Could you check a few things on this model? Use its own coordinates, in mm. Face numbers are marked on the shaded views. A direction names the side the tool comes from. Round coordinates to 2 decimals unless told otherwise and drop trailing zeros. Loops run counter-clockwise (first coordinate to the right, second up) from the corner with the lowest first, then second, coordinate; pieces in that order, holes last. Notation, with made-up numbers: (8, 71.25) -> (35, 71.25) arc R24 cw to (35, 101.25) -> close; hole circle Ø10 at (20.25, 55). An arc over 180 degrees is marked (long way). One line per item, written item: value.
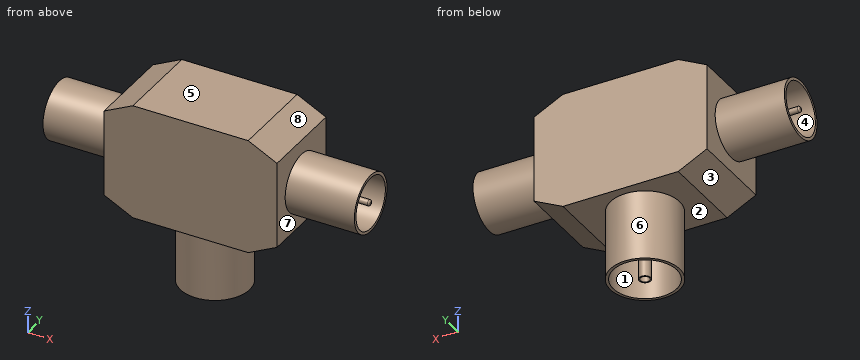
from build123d import *

# Parameters (mm, degrees)
BOSS_EXTRUDE1_DEPTH  = 15
SKETCH2_R            = 6
SKETCH2_R_2          = 5.5
BOSS_EXTRUDE2_DEPTH  = 12
SKETCH3_R            = 1
SKETCH3_R_2          = 0.8
BOSS_EXTRUDE3_DEPTH  = 12
SKETCH4_R            = 5
SKETCH4_R_2          = 4.5
SKETCH4_R_3          = 0.5
BOSS_EXTRUDE4_DEPTH  = 12
FILLET2_R            = 0.3
FILLET2_OF_MIRROR1_R = 0.3


with BuildPart() as part:
    # Sketch1 → Boss-Extrude1 (new body)
    with BuildSketch(Plane(origin=(0, 0, 0), x_dir=(1, 0, 0), z_dir=(0, 1, 0))):
        Polygon((10, 20), (15, 17.5), (15, 2.5), (10, 0), (-10, 0), (-15, 2.5), (-15, 17.5), (-10, 20), align=None)
    extrude(amount=BOSS_EXTRUDE1_DEPTH)

    # Sketch2 → Boss-Extrude2 (add)
    with BuildSketch(Plane(origin=(0, 0, -20), x_dir=(-1, 0, 0), z_dir=(0, 0, -1))):
        with Locations((0, 7.5)):
            Circle(SKETCH2_R)
        with Locations((0, 7.5)):
            Circle(SKETCH2_R_2, mode=Mode.SUBTRACT)
    extrude(amount=BOSS_EXTRUDE2_DEPTH)

    # Sketch3 → Boss-Extrude3 (add)
    with BuildSketch(Plane(origin=(0, 0, -20), x_dir=(-1, 0, 0), z_dir=(0, 0, -1))):
        with Locations((0, 7.5)):
            Circle(SKETCH3_R)
        with Locations((0, 7.5)):
            Circle(SKETCH3_R_2, mode=Mode.SUBTRACT)
    extrude(amount=BOSS_EXTRUDE3_DEPTH)

    # Sketch4 → Boss-Extrude4 (add)
    with BuildSketch(Plane.ZY.offset(15)):
        with Locations((-10, 7.5)):
            Circle(SKETCH4_R)
        with Locations((-10, 7.5)):
            Circle(SKETCH4_R_2, mode=Mode.SUBTRACT)
        with Locations((-10, 7.5)):
            Circle(SKETCH4_R_3)
    boss_extrude4 = extrude(amount=BOSS_EXTRUDE4_DEPTH)

    # Fillet2
    fillet2_edges = [part.edges().sort_by_distance(p)[0] for p in [
        (-27, 7.5, -10.5),
    ]]
    fillet(fillet2_edges, radius=FILLET2_R)

    # Mirror1: Boss-Extrude4 across plane
    add(boss_extrude4.mirror(Plane(origin=(0, 0, 0), x_dir=(0, 0, 1), z_dir=(1, 0, 0))))

    # Fillet2 of Mirror1
    fillet2_of_mirror1_edges = [part.edges().sort_by_distance(p)[0] for p in [
        (27, 7.5, -10.5),
    ]]
    fillet(fillet2_of_mirror1_edges, radius=FILLET2_OF_MIRROR1_R)


solid = part.part
(1) I'm going to push flat-ended pins straight in: pin 1 Ø1 at (y, z) = (7, -16.5) entering from -X; pin 2 Ø0.5 at (x, y) = (0, 7) entering from -Z; pin 3 Ø6 at (y, z) = (10, -28.5) entering from -X. Where does each tip first touch, or does it pass through?
Recorded:
pin 1: x = -15
pin 2: z = -20
pin 3: x = -6
(2) If we section it at D-D, the plane z = -4: Please give me the cut outline in (x, y).
Recorded:
outline: (-15, 0) -> (15, 0) -> (15, 15) -> (-15, 15) -> close
(3) If we section it at B-B, the plane x = -17.5: Please give me the cut outline in (y, z), then the cut area to 3 significant figures.
Recorded:
outline: circle Ø10 at (7.5, -10); circle Ø1 at (7.5, -10); hole circle Ø9 at (7.5, -10)
area: 15.7 mm²
(4) If we section it at A-A, the plane z = -23: Please give me the cut outline in (x, y), then the cut area to 3 significant figures.
Recorded:
outline: circle Ø12 at (0, 7.5); circle Ø2 at (0, 7.5); hole circle Ø11 at (0, 7.5); hole circle Ø1.6 at (0, 7.5)
area: 19.2 mm²
(5) If I drill on L1, parallel to Y at x = -22.25, z = -10; L2, parallel to Y at x = 0, z = -23.5; L3, parallel to X at y = 8, z = -27.5, over which ranges is the centre line in solid material (lowest first)?
Recorded:
L1: 2.5 to 3, 7 to 8, 12 to 12.5
L2: 1.5 to 2, 6.5 to 6.7, 8.3 to 8.5, 13 to 13.5
L3: -5.98 to -5.48, -0.87 to -0.62, 0.62 to 0.87, 5.48 to 5.98
(6) If we section it at C-C, the plane x = 0: Please give me the cut outline in (y, z), then the cut area to 3 significant figures.
Recorded:
outline: (0, -20) -> (1.5, -20) -> (1.5, -32) -> (2, -32) -> (2, -20) -> (6.5, -20) -> (6.5, -32) -> (6.7, -32) -> (6.7, -20) -> (8.3, -20) -> (8.3, -32) -> (8.5, -32) -> (8.5, -20) -> (13, -20) -> (13, -32) -> (13.5, -32) -> (13.5, -20) -> (15, -20) -> (15, 0) -> (0, 0) -> close
area: 317 mm²
(7) Thinking about a two-plate mould opening in X: for the marked faces 1, 2 and 3, which applies, released by +X, released by -X, zero draft, split by the parting line, or undercut?
Recorded:
face 1: undercut
face 2: zero draft
face 3: released by -X
(8) For the marked faces 4, 5, 6, 7 and 8, which set-ups out of +Z, -Z, +X, -X, +Y, -Y let a thin tool reach every point of the face, with its end or its side?
Recorded:
face 4: -X
face 5: +Z, +X, -X, +Y, -Y
face 6: -Z
face 7: +X
face 8: +Z, +X, +Y, -Y
